Could you check a few things on this model? Use its own coordinates, in mm. Face numbers are marked on the shaded views. A direction names the side the tool comes from. Round coordinates to 2 decimals unless told otherwise and drop trailing zeros. Loops run counter-clockwise (first coordinate to the right, second up) from the corner with the lowest first, then second, coordinate; pieces in that order, holes last. Notation, with made-up numbers: (-7.5, 55) -> (23.5, 55) arc R22 ccw to (23.5, 61) -> close; hole circle Ø4 at (57, 34.5). An arc over 180 degrees is marked (long way). Write each question's results on one line, items separated by ' | '.
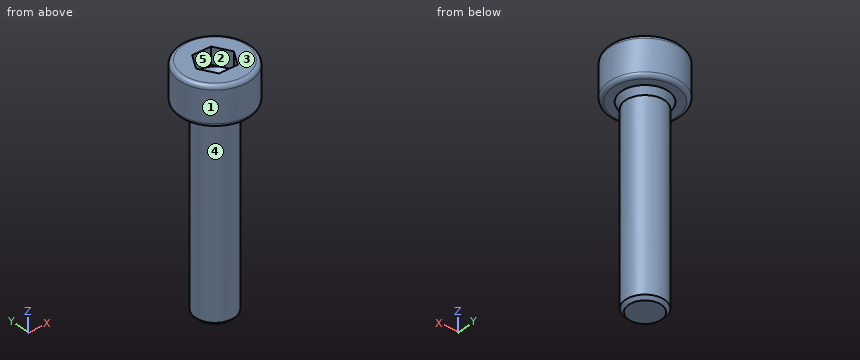
Solid Edge part; units mm, degrees
sketch "Sketch1" plane through (0, 0, 0) normal (0, -1, 0) x (1, 0, 0)
  line L0 (2.75, 3) -> (2.75, 0)
  line L1 (2.75, 0) -> (1.8, 0)
  line L2 (1.8, 0) -> (1.5, -0.5196)
  line L3 (1.5, -0.5196) -> (1.5, -15)
  line L4 (1.5, -15) -> (0, -15)
  line L5 (1.25, 1.7) -> (0, 0.9783)
  line L6 (1.25, 3) -> (1.25, 1.7)
  line L7 (2.75, 3) -> (1.25, 3)
revolve "RevolvedProtrusion1" add sketch "Sketch1" angle 360 about axis through (0, 0, -6) along (0, 0, 1)
cosmetic_thread "Thread1"
chamfer "Chamfer_1" distance 0.25 angle 45 1 edges at (-1.5, 0, -15)
fillet "Round_1" radius 0.3 2 edges at (-2.75, 0, 0) (-2.75, 0, 3)
sketch "Sketch2" plane through (0, 0, 3) normal (0, 0, 1) x (0, 1, 0)
  line L0 (-1.25, 0.7217) -> (-1.25, -0.7217)
  line L1 (0, -1.4434) -> (-1.25, -0.7217)
  line L2 (1.25, -0.7217) -> (0, -1.4434)
  line L3 (1.25, 0.7217) -> (1.25, -0.7217)
  line L4 (0, 1.4434) -> (1.25, 0.7217)
  line L5 (-1.25, 0.7217) -> (0, 1.4434)
extrude "Cutout1" cut sketch "Sketch2" against normal up to vertex (1.3 mm away)
properties material "Galvanized steel"
1) If we mould it in two halves opening along Y, with no side actions, what happens to the marked faces 3, 4 and 5? For each: released by +Y, released by -Y, zero draft, split by the parting line, or undercut.
Model answer:
face 3: zero draft | face 4: split by the parting line | face 5: undercut
2) I want a section at A-A, the plane z = -11.25. Write out the boundary of the cut face in (x, y), plus the area to 3 significant figures.
Model answer:
outline: circle Ø3 at (0, 0) | area: 7.07 mm2
3) For the marked faces 1 and 2, which set-ups out of +Z, -Z, +X, -X, +Y, -Y let a thin tool reach every point of the face, with its end or its side?
Model answer:
face 1: +Z, -Z | face 2: +Z
4) I need wall thicknesses on line 1 (Z direction, x = 1.75, y = 1.15); line 2 (X direction, y = 0.1, z = 1.25); line 3 (Y direction, x = -0.1, z = -10). Which ranges of each line are inside material? Lowest first, please.
Model answer:
line 1: z = 0 to 3 | line 2: x = -2.75 to -0.46, 0.46 to 2.75 | line 3: y = -1.5 to 1.5
5) I'm going to push flat-ended pins straight in: pin 1 (3 mm diameter, centred on x = -1.5, z = -6, fed in from +Y); pin 2 (3 mm diameter, centred on y = -0.5, z = -12.5, fed in from +X). Where does each tip first touch, or does it pass through?
Model answer:
pin 1: stops at y = 1.5 | pin 2: stops at x = 1.5
